Input: part model. Units: mm. Frame: model coordinates. Face numbers are marked on the shaded views. A direction names the side the tool comes from. Give positions to 0.01 mm unless a question says otherwise; leave off trailing zeros. Loops run counter-clockwise (first coordinate to the right, second up) from the corner with the lowest first, then second, coordinate; pieces in that order, holes last. Notation, with made-up numbers: (-32.75, 55) - (4.25, 55) arc R23 ccw to (4.25, 93) - close; hole circle Ø11 at (66, 10). An arc over 180 degrees is marked (long way). Answer as a JSON object with one key per item and string values. Group by question number.
(1) Access query for the marked faces 5, 6 and 7. Directions: +Z, -Z, +X, -X, +Y, -Y. A direction counts if a zero-diameter tool reaches every point of the face in a straight line with its end or side. Return the directions, or none.
(2) Section query D-D (y = -57.5). Return loops of the section in (x, z), plus the area to 3 significant figures.
(3) Section query C-C (y = -82.5). Return loops of the section in (x, z), plus the area to 3 significant figures.
(4) Section query A-A (z = 48). Return loops of the section in (x, y), plus the area to 3 significant figures.
(5) Section query B-B (x = 0). Return loops of the section in (y, z).
(6) Pin query (flat end, axial travel): P1, Ø10, axis at x = -9, y = -51.5, coming from the -Z side; P2, Ø8, axis at x = 0, y = -102.5, coming from the +Z side; P3, Ø6, axis at y = -87, z = 12.5, coming from the +X side; P4, Ø8, axis at x = -26, z = 33.5, coming from the -Y side. Return the tip coordinate at first contact, or that it passes through.
(7) Material intervals for L1, parallel to Z at x = -35.5, y = -21.5; L2, parallel to Y at x = 0, z = 41; L3, parallel to Z at x = -10.5, y = -69, sorted ascending.
(8) Mould query, pull axis X, two halves, no side actions, for the marked faces 1, 2, 3 and 4. Classes: +X half, -X half, draft (parallel to the pull), parting line (faces both ways), or undercut.
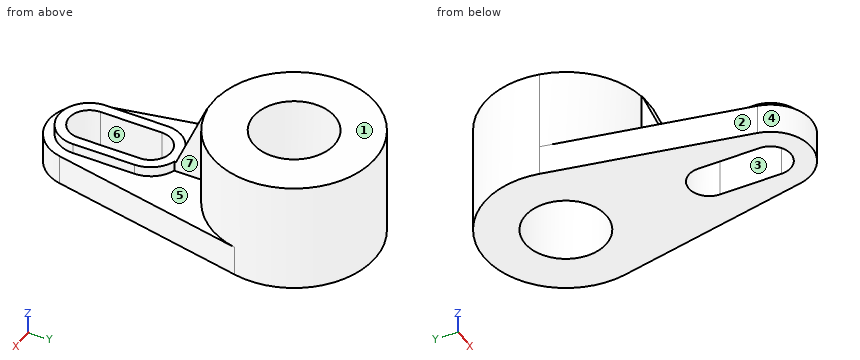
```python
from build123d import *

# Parameters (mm, degrees)
BOSS_EXTRUDE1_DEPTH = 15
BOSS_EXTRUDE2_DEPTH = 20
SKETCH1_4_R         = 40
SKETCH1_4_R_2       = 20
BOSS_EXTRUDE3_DEPTH = 55
BOSS_EXTRUDE6_DEPTH = 5


with BuildPart() as part:
    # Sketch1 → Boss-Extrude1 (new body)
    with BuildSketch(Plane(origin=(0, 0, 0), x_dir=(0, 1, 0), z_dir=(0, 0, 1))):
        with BuildLine():
            Line((-8, 39.191835885), (-104, 19.595917942))
            ThreePointArc((-104, 19.595917942), (-120, 0), (-104, -19.595917942))
            Line((-104, -19.595917942), (-8, -39.191835885))
            ThreePointArc((-8, -39.191835885), (-40, 0), (-8, 39.191835885))
        make_face()
        with BuildLine():
            ThreePointArc((-100, -15), (-115, 0), (-100, 15))
            Line((-100, 15), (-70, 15))
            ThreePointArc((-70, 15), (-55, 0), (-70, -15))
            Line((-70, -15), (-100, -15))
        make_face(mode=Mode.SUBTRACT)
    extrude(amount=BOSS_EXTRUDE1_DEPTH)

    # Sketch1_3 → Boss-Extrude2 (add)
    with BuildSketch(Plane(origin=(0, 0, 0), x_dir=(0, 1, 0), z_dir=(0, 0, 1))):
        with BuildLine():
            Line((-100, 15), (-70, 15))
            ThreePointArc((-70, 15), (-55, 0), (-70, -15))
            Line((-70, -15), (-100, -15))
            ThreePointArc((-100, -15), (-115, 0), (-100, 15))
        make_face()
        with BuildLine():
            ThreePointArc((-70, -10), (-60, 0), (-70, 10))
            Line((-70, 10), (-100, 10))
            ThreePointArc((-100, 10), (-110, 0), (-100, -10))
            Line((-100, -10), (-70, -10))
        make_face(mode=Mode.SUBTRACT)
    extrude(amount=BOSS_EXTRUDE2_DEPTH)

    # Sketch1_4 → Boss-Extrude3 (add)
    with BuildSketch(Plane(origin=(0, 0, 0), x_dir=(0, 1, 0), z_dir=(0, 0, 1))):
        with Locations(Location((0, 0, 0), (0, 0, 101.536959033))):
            Circle(SKETCH1_4_R)
        with Locations(Location((0, 0, 0), (0, 0, 270))):
            Circle(SKETCH1_4_R_2, mode=Mode.SUBTRACT)
    extrude(amount=BOSS_EXTRUDE3_DEPTH)

    # Sketch2 → Boss-Extrude6 (add, symmetric)
    with BuildSketch(Plane.YZ):
        Polygon((-55, 20), (-40, 55), (-39, 55), (-39, 15), (-56, 15), (-56, 20), align=None)
    extrude(amount=BOSS_EXTRUDE6_DEPTH, both=True)


solid = part.part
```
Recorded:
{
 "1": {"face 5": "+Z", "face 6": "+Z, -Z", "face 7": "+Z, +X"},
 "2": {"outline": "(-29.09, 0) - (29.09, 0) - (29.09, 15) - (8.29, 15) - (8.29, 20) - (-8.29, 20) - (-8.29, 15) - (-29.09, 15) - close", "area": "956 mm^2"},
 "3": {"outline": "(-23.98, 0) - (-10, 0) - (-10, 20) - (-15, 20) - (-15, 15) - (-23.98, 15) - close; (10, 0) - (23.98, 0) - (23.98, 15) - (15, 15) - (15, 20) - (10, 20) - close", "area": "470 mm^2"},
 "4": {"outline": "(-5, -43) - (5, -43) - (5, -39.69) arc R40 ccw (long way) to (-5, -39.69) - close; hole circle Ø40 at (0, 0)", "area": "3,800 mm^2"},
 "5": {"outline": "(-120, 0) - (-110, 0) - (-110, 20) - (-115, 20) - (-115, 15) - (-120, 15) - close; (-60, 0) - (-20, 0) - (-20, 55) - (-40, 55) - (-55, 20) - (-60, 20) - close; (20, 0) - (40, 0) - (40, 55) - (20, 55) - close"},
 "6": {"P1": "stops at z = 0", "P2": "passes through", "P3": "stops at x = 23.68", "P4": "stops at y = -33.41"},
 "7": {"L1": "z = 0 to 15", "L2": "y = -46 to -20, 20 to 40", "L3": "z = 0 to 20"},
 "8": {"face 1": "draft", "face 2": "-X half", "face 3": "undercut", "face 4": "parting line"}
}
